Could you check a few things on this model? Use its own coordinates, in mm. A direction names the side the tool comes from. Give positions to 0.01 mm unless a question says otherwise; leave off trailing zeros. Write each loop counter-clockwise with the first axis right and the second up, starting at its lowest first coordinate (ties: lowest second). Pieces come first, ordered by that corner, then holes. Notation, with made-up numbers: M 50.25,17.5 L 76.25,17.5 A21 ccw 76.25,26.5 Z; hole C 23,37 d5. An arc over 180 degrees is marked long. Answer as a JSON object with one key per item and string values. Group by question number.
Autodesk Inventor part; units mm, degrees
ref_plane "YZ Plane" through (0, 0, 0) normal (1, 0, 0) x (0, 1, 0)
ref_plane "XZ Plane" through (0, 0, 0) normal (0, 1, 0) x (-1, 0, 0)
ref_plane "XY Plane" through (0, 0, 0) normal (0, 0, 1) x (1, 0, 0)
sketch "Sketch1" plane through (0, 0, 0) normal (0, 0, 1) x (1, 0, 0)
  line L0 (0, 0) -> (-304.8, 0)
  line L1 (-304.8, 0) -> (-304.8, 25.4)
  line L2 (-304.8, 25.4) -> (0, 25.4)
  line L3 (0, 25.4) -> (0, 0)
  dimension "d0" = 25.4
  dimension "d1" = 304.8
extrude "Extrusion1" add sketch "Sketch1" along normal blind 25.4
shell "Shell1" thickness 1.5875 removed faces 2 at (0, 16.9333, 8.4667) at (-304.8, 8.4667, 8.4667)
sketch "Sketch2" plane through (0, 0, 25.4) normal (0, 0, 1) x (1, 0, 0)
  line L0 (0, 0) -> (-304.8, 0)
  line L1 (0, 25.4) -> (0, 0)
  circle A0 centre (-12.7, 12.7) radius 3.175
  dimension "d5" = 12.7
  dimension "d6" = 12.7
  dimension "d7" = 6.35
extrude "Extrusion2" cut sketch "Sketch2" against normal through all
fillet "Fillet1" radius 12.7 2 edges at (0, 25.4, 12.7) (0, 0, 12.7)
properties part number "Shovel_Arm" material "Aluminum-6061"
1) If we section it at A-A, the plane z = 16.75: List the corners of the cut face in (x, y) for me.
2) For faces 1 (the flat face through (-161, 25.4, 13)), 2 (the flat face through (-154, 1.588, 13)), which set-ups out of +Z, -Z, +X, -X, +Y, -Y let a thin tool reach every point of the face, with its end or its side?
3) If we section it at C-C, the plane y = 12.7: List the corners of the cut face in (x, z) for me (1 decimal), plus the area to 3 significant figures.
4) We'd pull the mould along Z, two halves only. Please class faces 3 (the cylindrical face through (-11.2, 9.9, 24.6)), 4 (the flat face through (-155, 13, 25.4)), 5 (the flat face through (-155, 13, 23.812)): released by +Z, released by -Z, zero draft, split by the parting line, or undercut.
5) Please list where these lines run through material, in increasing order: line 1 along Z through (x, y) = (-130.5, 13.5); line 2 along Y through (x, z) = (-12.7, 1.15) (3 decimals). Write a range as from..to.
6) I'm going to push a flat-ended pin straight in: pin 1 (5 mm diameter, centred on y = 20, z = 21.5, fed in from +X). Where does the tip first touch, or does it pass through?
7) If we section it at B-B, the plane x = -124.5: List the corners of the cut face in (y, z) for me, plus the area to 3 significant figures.
Taken from the geometry:
{
 "1": {"outline": "M -304.8,0 L -12.7,0 A12.7 ccw -6.55,1.59 L -304.8,1.59 Z; M -304.8,23.81 L -6.55,23.81 A12.7 ccw -12.7,25.4 L -304.8,25.4 Z"},
 "2": {"face 1": "+Z, -Z, +X, -X, +Y", "face 2": "+X, -X"},
 "3": {"outline": "M -304.8,0 L -15.9,0 L -15.9,1.6 L -304.8,1.6 Z; M -304.8,23.8 L -15.9,23.8 L -15.9,25.4 L -304.8,25.4 Z; M -9.5,0 L 0,0 L 0,1.6 L -9.5,1.6 Z; M -9.5,23.8 L 0,23.8 L 0,25.4 L -9.5,25.4 Z", "area": "948 mm²"},
 "4": {"face 3": "zero draft", "face 4": "released by +Z", "face 5": "undercut"},
 "5": {"line 1": "0..1.59, 23.81..25.4", "line 2": "0..9.525, 15.875..25.4"},
 "6": {"pin 1": "x = -1.7"},
 "7": {"outline": "M 0,0 L 25.4,0 L 25.4,25.4 L 0,25.4 Z; hole M 1.59,1.59 L 23.81,1.59 L 23.81,23.81 L 1.59,23.81 Z", "area": "151 mm²"}
}
